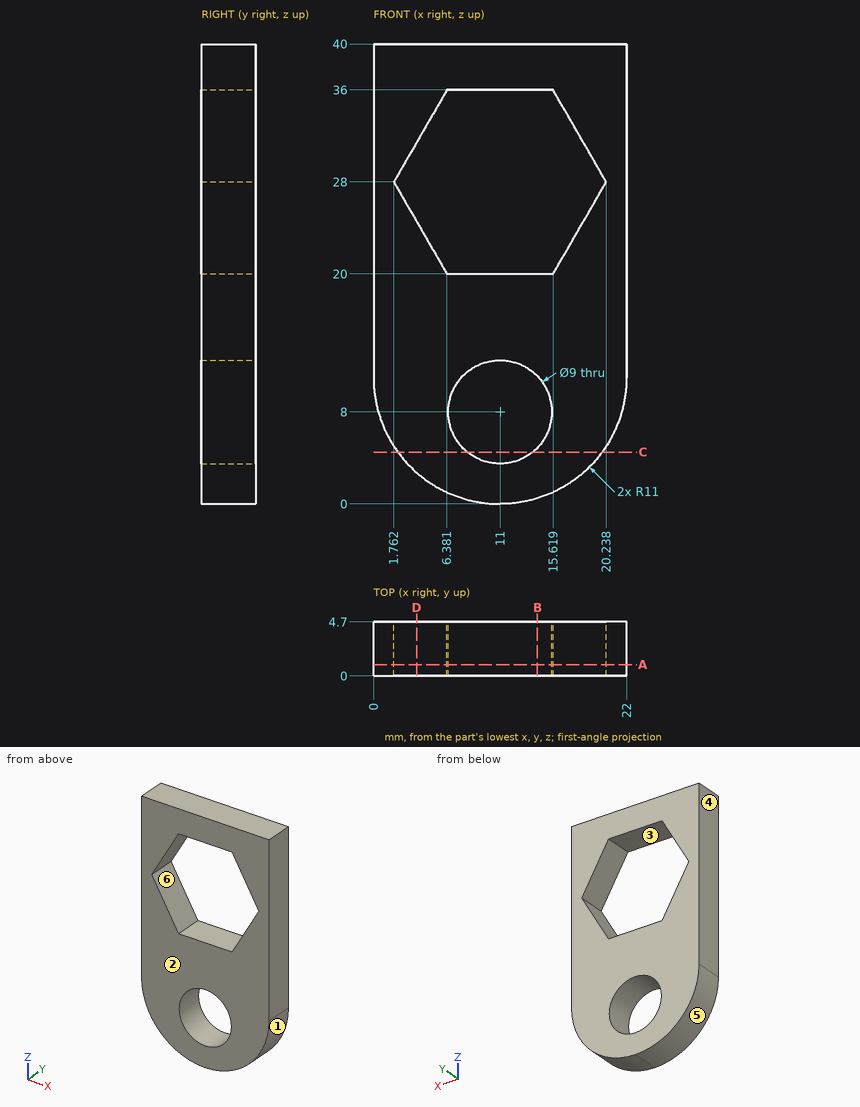
For this review, use the dimensioned drawing (mm, ordinates from the lowest corner) and the shaded views. A direction names the side the tool comes from. Coordinates: 2 decimals unless noted, no trailing zeros. Loops run counter-clockwise (first coordinate to the right, second up) from the corner with the lowest first, then second, coordinate; pieces in that order, holes last. Notation, with made-up numbers: (20.5, -37) - (53.5, -37) arc R29 cw to (53.5, -17) - close; hole circle Ø5 at (-14.5, 38.5). An arc over 180 degrees is marked (long way). Use one line per item in the form item = value. Start each with the question number.
1) Take a section at A-A (y = 1). State how many separate pieces and enclosed holes the cut face has, plus the area to 3 significant figures.
2) Take a section at C-C (z = 4.5). State the section outline as (x, y) points.
3) For pin 1 (12 mm diameter, centred on x = 5.5, z = 21, fed in from -Y); pin 2 (8 mm diameter, centred on x = 11, z = 8, fed in from -Y), all flat-tipped, find the tip position at first contact; note any pin that passes through.
4) Draft analysis for pull direction X (two halves, no side actions). For the marked faces 1, 2, 3 and 4, state which applies: released by +X, released by -X, zero draft, split by the parting line, or undercut.
5) Take a section at D-D (x = 3.75). State the section outline as (y, z) points, plus the area to 3 significant figures.
6) For the marked faces 5 and 6, list the 3-axis set-ups (+Z, -Z, +X, -X, +Y, -Y) from which the entire face can be reached by the end or side of a thin tool; tool diameter is ignored.
7) To check wall thickness, follow probe 1 along Z at (x, y) = (11, 2.5); probe 2 along Z at (x, y) = (8, 1.5) (1 decimal); probe 3 along X at (y, z) = (1.9, 8). State the ranges of each line that lie inside material, in increasing order. Write a range as from..to.
8) Take a section at B-B (x = 14.25). State the section outline as (y, z) points.
From the geometry:
q1.separate_pieces = 1
q1.enclosed_holes = 2
q1.area = 543 mm2
q2.outline = (2.13, 0) - (8.17, 0) - (8.17, 4.7) - (2.13, 4.7) - close; (13.83, 0) - (19.87, 0) - (19.87, 4.7) - (13.83, 4.7) - close
q3.pin_1 = 0
q3.pin_2 = through
q4.face_1 = released by +X
q4.face_2 = zero draft
q4.face_3 = undercut
q4.face_4 = released by -X
q5.outline = (0, 2.73) - (4.7, 2.73) - (4.7, 24.56) - (0, 24.56) - close; (0, 31.44) - (4.7, 31.44) - (4.7, 40) - (0, 40) - close
q5.area = 143 mm2
q6.face_5 = -Z, -X, +Y, -Y
q6.face_6 = +Y, -Y
q7.probe_1 = 0..3.5, 12.5..20, 36..40
q7.probe_2 = 0.4..4.6, 11.4..20, 36..40
q7.probe_3 = 0.42..6.5, 15.5..21.58
q8.outline = (0, 0.49) - (4.7, 0.49) - (4.7, 4.89) - (0, 4.89) - close; (0, 11.11) - (4.7, 11.11) - (4.7, 20) - (0, 20) - close; (0, 36) - (4.7, 36) - (4.7, 40) - (0, 40) - close
